Here's how the part is built. I have some questions about the finished solid (model axes, mm). Face numbers are marked on the shaded views. A direction names the side the tool comes from. Round coordinates to 2 decimals unless told otherwise and drop trailing zeros. Write each loop counter-clockwise with the first axis right and the second up, starting at its lowest first coordinate (ties: lowest second). Pieces come first, ordered by that corner, then holes. Notation, with made-up numbers: (27.25, -21.75) -> (78.25, -21.75) arc R26 cw to (78.25, -7.75) -> close; hole circle Ø6 at (14.25, 25). An arc over 180 degrees is marked (long way). Answer in a Markdown table with one row per item.
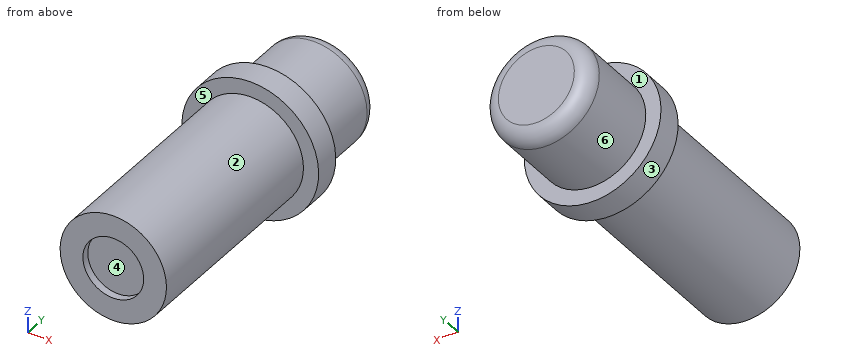
from build123d import *

# Parameters (mm, degrees)
SKETCH1_R           = 3.5
BOSS_EXTRUDE1_DEPTH = 14
BOSS_EXTRUDE2_START = 14
SKETCH1_4_R         = 4.5
BOSS_EXTRUDE2_DEPTH = 1.75
BOSS_EXTRUDE3_START = 15.75
SKETCH1_5_R         = 3.5
BOSS_EXTRUDE3_DEPTH = 5.75
FILLET1_R           = 1
SKETCH2_R           = 2
CUT_EXTRUDE1_DEPTH  = 0.5


with BuildPart() as part:
    # Sketch1 → Boss-Extrude1 (new body)
    with BuildSketch(Plane(origin=(0, 0, 0), x_dir=(1, 0, 0), z_dir=(0, 1, 0))):
        with Locations(Location((0, 0, 0), (0, 0, 270))):
            Circle(SKETCH1_R)
    extrude(amount=BOSS_EXTRUDE1_DEPTH)

    # Sketch1<4> → Boss-Extrude2 (add)
    with BuildSketch(Plane(origin=(0, 0, 0), x_dir=(1, 0, 0), z_dir=(0, 1, 0)).offset(BOSS_EXTRUDE2_START)):
        with Locations(Location((0, 0, 0), (0, 0, 270))):
            Circle(SKETCH1_4_R)
    extrude(amount=BOSS_EXTRUDE2_DEPTH)

    # Sketch1<5> → Boss-Extrude3 (add)
    with BuildSketch(Plane(origin=(0, 0, 0), x_dir=(1, 0, 0), z_dir=(0, 1, 0)).offset(BOSS_EXTRUDE3_START)):
        with Locations(Location((0, 0, 0), (0, 0, 270))):
            Circle(SKETCH1_5_R)
    extrude(amount=BOSS_EXTRUDE3_DEPTH)

    # Fillet1
    fillet1_edges = [part.edges().sort_by_distance(p)[0] for p in [
        (0, 21.5, -3.5),
    ]]
    fillet(fillet1_edges, radius=FILLET1_R)

    # Sketch2 → Cut-Extrude1 (cut)
    with BuildSketch(Plane.XZ):
        with Locations(Location((0, 0, 0), (0, 0, 270))):
            Circle(SKETCH2_R)
    extrude(amount=-CUT_EXTRUDE1_DEPTH, mode=Mode.SUBTRACT)


solid = part.part
1) For pin 1 (5 mm diameter, centred on x = 2.5, y = 19, fed in from +Z); pin 2 (4 mm diameter, centred on y = 4, z = -1.5, fed in from -X); pin 3 (3 mm diameter, centred on x = 2, y = 18.5, fed in from -Z), each with a flat end and sliding along its axis, tell me the tip position at first contact or that it passes through.
Response:
| item | result |
|---|---|
| pin 1 | stops at z = 3.5 |
| pin 2 | stops at x = -3.5 |
| pin 3 | stops at z = -3.46 |
2) I need wall thicknesses on line 1 (X direction, y = 0.25, z = 0); line 2 (Y direction, x = -2.75, z = -3); line 3 (Y direction, x = 0.25, z = -1.75). Which ranges of each line are inside material? Lowest first, please. Write a range as [from, to].
Response:
| item | result |
|---|---|
| line 1 | x = [-3.5, -2], [2, 3.5] |
| line 2 | y = [14, 15.75] |
| line 3 | y = [0.5, 21.5] |
3) I want a section at B-B, the plane z = 0. List the corners of the cut face in (x, y) for me, and give its area (3 significant figures).
Response:
| item | result |
|---|---|
| outline | (-4.5, 14) -> (-3.5, 14) -> (-3.5, 0) -> (-2, 0) -> (-2, 0.5) -> (2, 0.5) -> (2, 0) -> (3.5, 0) -> (3.5, 14) -> (4.5, 14) -> (4.5, 15.75) -> (3.5, 15.75) -> (3.5, 20.5) arc R1 ccw to (2.5, 21.5) -> (-2.5, 21.5) arc R1 ccw to (-3.5, 20.5) -> (-3.5, 15.75) -> (-4.5, 15.75) -> close |
| area | 152 mm^2 |
4) I want a section at A-A, the plane x = 0. List the corners of the cut face in (y, z) for me.
Response:
| item | result |
|---|---|
| outline | (0, -3.5) -> (14, -3.5) -> (14, -4.5) -> (15.75, -4.5) -> (15.75, -3.5) -> (20.5, -3.5) arc R1 ccw to (21.5, -2.5) -> (21.5, 2.5) arc R1 ccw to (20.5, 3.5) -> (15.75, 3.5) -> (15.75, 4.5) -> (14, 4.5) -> (14, 3.5) -> (0, 3.5) -> (0, 2) -> (0.5, 2) -> (0.5, -2) -> (0, -2) -> close |
5) Which directions (+Z, -Z, +X, -X, +Y, -Y) give clear straight access to the entire face, cutting with the end or side of a thin tool? Please do the marked faces 1, 2 and 3.
Response:
| item | result |
|---|---|
| face 1 | +Y |
| face 2 | -Y |
| face 3 | +Y, -Y |
6) I want a section at C-C, the plane y = 5.25. List the corners of the cut face in (x, z) for me, and give its area (3 significant figures).
Response:
| item | result |
|---|---|
| outline | circle Ø7 at (0, 0) |
| area | 38.5 mm^2 |
7) We'd pull the mould along X, two halves only. Please class the marked faces 4, 5 and 6: +X half, -X half, draft (parallel to the pull), parting line (faces both ways), or undercut.
Response:
| item | result |
|---|---|
| face 4 | undercut |
| face 5 | draft |
| face 6 | parting line |
